from build123d import *

# Parameters (mm, degrees)
SKETCH_R  = 3
PAD_DEPTH = 4


with BuildPart() as part:
    # Sketch → Pad (new body)
    with BuildSketch(Plane.XY):
        with BuildLine():
            Line((-78, -10), (-78, -119.313708))
            ThreePointArc((-78, -119.313708), (-76.765367, -121.161468), (-74.585786, -120.727922))
            Line((-74.585786, -120.727922), (-58.585786, -104.727922))
            ThreePointArc((-58.585786, -104.727922), (-58.152241, -104.079075), (-58, -103.313708))
            Line((-58, -58), (-58, -103.313708))
            ThreePointArc((-57.414214, -56.585786), (-57.847759, -57.234633), (-58, -58))
            Line((-57.414214, -56.585786), (-19.414214, -18.585786))
            ThreePointArc((-18, -18), (-18.765367, -18.152241), (-19.414214, -18.585786))
            Line((-18, -18), (18, -18))
            ThreePointArc((19.414214, -18.585786), (18.765367, -18.152241), (18, -18))
            Line((19.414214, -18.585786), (57.414214, -56.585786))
            ThreePointArc((58, -58), (57.847759, -57.234633), (57.414214, -56.585786))
            Line((58, -58), (58, -103.313708))
            ThreePointArc((58, -103.313708), (58.152241, -104.079075), (58.585786, -104.727922))
            Line((58.585786, -104.727922), (74.585786, -120.727922))
            ThreePointArc((74.585786, -120.727922), (76.765367, -121.161468), (78, -119.313708))
            Line((78, -119.313708), (78, -10))
            Line((57.5, -10), (78, -10))
            Line((57.5, -3), (57.5, -10))
            Line((57.5, -3), (-57.5, -3))
            Line((-57.5, -10), (-57.5, -3))
            Line((-78, -10), (-57.5, -10))
        make_face()
        with Locations((-68, -100)):
            Circle(SKETCH_R, mode=Mode.SUBTRACT)
        with Locations((68, -100)):
            Circle(SKETCH_R, mode=Mode.SUBTRACT)
        with Locations((-68, -20)):
            Circle(SKETCH_R, mode=Mode.SUBTRACT)
        with Locations((68, -20)):
            Circle(SKETCH_R, mode=Mode.SUBTRACT)
    extrude(amount=PAD_DEPTH)


solid = part.part
Input: part model. Units: mm. Frame: model coordinates. A direction names the side the tool comes from. Round coordinates to 2 decimals unless told otherwise and drop trailing zeros. Write each loop counter-clockwise with the first axis right and the second up, starting at its lowest first coordinate (ties: lowest second). Pieces come first, ordered by that corner, then holes.
1) Cut plane D-D (y = -38.5). Return the cut outline in (x, z).
2) Cut plane A-A (y = -92). Return the cut outline in (x, z).
3) Draft query along X for faces 4 (the flat face through (57.5, -6, 2)), 5 (the flat face through (1, -3, 2)), 6 (the cylindrical face through (65.6, -21.8, 2)), 7 (the cylindrical face through (-70.4, -21.8, 2)). Return one class per face: pulls with the +X half, pulls with the -X half, needs draft (parallel to the pull), parting line crosses it, or undercut.
4) Cut plane C-C (x = 68). Return the cut outline in (y, z), then the cut area to 3 significant figures.
5) Cut plane B-B (z = 2.4). Return the cut outline in (x, y), then the cut area to 3 significant figures.
6) Reachability of faces 1 (the flat face through (-68, -10, 2)), 2 (the flat face through (-66.7, -112.84, 1.97)), 3 (the flat face through (68, -10, 2)) from +Z, -Z, +X, -X, +Y, -Y: full face, straight path, thin tool, end or side. Return the list, or none.
7) Ray query, L1, parallel to X at y = -59, z = 1.85; L2, parallel to Y at x = 68, z = 1.65; L3, parallel to X at y = -8.5, z = 2.4. Return the intervals inside material, ascending.
8) Contact query for a flat-ended pin moving along its axis: P1, Ø2, axis at x = -63.5, z = 2, coming from the +Y side. Output: stop coordinate, or through.
Geometry says:
1. outline: (-78, 0) - (-39.33, 0) - (-39.33, 4) - (-78, 4) - close; (39.33, 0) - (78, 0) - (78, 4) - (39.33, 4) - close
2. outline: (-78, 0) - (-58, 0) - (-58, 4) - (-78, 4) - close; (58, 0) - (78, 0) - (78, 4) - (58, 4) - close
3. face 4: pulls with the +X half
3. face 5: needs draft
3. face 6: undercut
3. face 7: undercut
4. outline: (-114.14, 0) - (-103, 0) - (-103, 4) - (-114.14, 4) - close; (-97, 0) - (-23, 0) - (-23, 4) - (-97, 4) - close; (-17, 0) - (-10, 0) - (-10, 4) - (-17, 4) - close
4. area: 369 mm2
5. outline: (-78, -119.31) arc R2 ccw to (-74.59, -120.73) - (-58.59, -104.73) arc R2 ccw to (-58, -103.31) - (-58, -58) arc R2 cw to (-57.41, -56.59) - (-19.41, -18.59) arc R2 cw to (-18, -18) - (18, -18) arc R2 cw to (19.41, -18.59) - (57.41, -56.59) arc R2 cw to (58, -58) - (58, -103.31) arc R2 ccw to (58.59, -104.73) - (74.59, -120.73) arc R2 ccw to (78, -119.31) - (78, -10) - (57.5, -10) - (57.5, -3) - (-57.5, -3) - (-57.5, -10) - (-78, -10) - close; hole circle Ø6 at (-68, -100); hole circle Ø6 at (-68, -20); hole circle Ø6 at (68, -100); hole circle Ø6 at (68, -20)
5. area: 7,310 mm2
6. face 1: +Z, -Z, -X, +Y
6. face 2: +Z, -Z, -Y
6. face 3: +Z, -Z, +X, +Y
7. L1: x = -78 to -58, 58 to 78
7. L2: y = -114.14 to -103, -97 to -23, -17 to -10
7. L3: x = -57.5 to 57.5
8. P1: stops at y = -10
